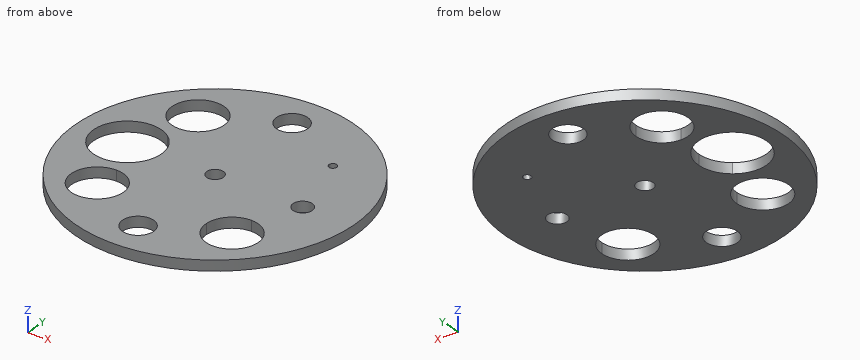
```python
from build123d import *

# Parameters (mm, degrees)
F0_R     = 26.75
F0_R_2   = 3
F0_R_3   = 1.85
F0_R_4   = 1.6
F1_DEPTH = 2


with BuildPart() as f1:
    # F0 (on Top) → F1 (new body)
    with BuildSketch(Plane.XY):
        Circle(F0_R)
        with Locations((0, -20)):
            Circle(F0_R_2, mode=Mode.SUBTRACT)
        with BuildLine():
            ThreePointArc((-13.081475, 8.081475), (-16.617009, 16.617009), (-8.081475, 13.081475))
            Line((-8.081475, 13.081475), (12.331475, 13.081475))
            ThreePointArc((12.331475, 13.081475), (13.081475, 13.831475), (13.831475, 13.081475))
            ThreePointArc((13.831475, 13.081475), (13.611806, 12.551145), (13.081475, 12.331475))
            Line((13.081475, 12.331475), (13.081475, -8.081475))
            ThreePointArc((13.081475, -8.081475), (16.617009, -9.545942), (18.081475, -13.081475))
            ThreePointArc((18.081475, -13.081475), (13.081475, -18.081475), (8.081475, -13.081475))
            Line((8.081475, -13.081475), (-8.081475, -13.081475))
            ThreePointArc((-8.081475, -13.081475), (-16.617009, -16.617009), (-13.081475, -8.081475))
            Line((-13.081475, -8.081475), (-13.081475, -5.186055))
            ThreePointArc((-13.081475, -5.186055), (-23.5, 0), (-13.081475, 5.186055))
            Line((-13.081475, 5.186055), (-13.081475, 8.081475))
        make_face(mode=Mode.SUBTRACT)
        with Locations((17, 0)):
            Circle(F0_R_3, mode=Mode.SUBTRACT)
        with Locations((0, 20)):
            Circle(F0_R_2, mode=Mode.SUBTRACT)
        with BuildLine():
            Line((12.331475, 13.081475), (-8.081475, 13.081475))
            ThreePointArc((-8.081475, 13.081475), (-9.545942, 9.545942), (-13.081475, 8.081475))
            Line((-13.081475, 8.081475), (-13.081475, 5.186055))
            ThreePointArc((-13.081475, 5.186055), (-11.181048, 2.896514), (-10.5, 0))
            ThreePointArc((-10.5, 0), (-11.181048, -2.896514), (-13.081475, -5.186055))
            Line((-13.081475, -5.186055), (-13.081475, -8.081475))
            ThreePointArc((-13.081475, -8.081475), (-9.545942, -9.545942), (-8.081475, -13.081475))
            Line((-8.081475, -13.081475), (8.081475, -13.081475))
            ThreePointArc((8.081475, -13.081475), (9.545942, -9.545942), (13.081475, -8.081475))
            Line((13.081475, -8.081475), (13.081475, 12.331475))
            ThreePointArc((13.081475, 12.331475), (12.551145, 12.551145), (12.331475, 13.081475))
        make_face()
        Circle(F0_R_4, mode=Mode.SUBTRACT)
    extrude(amount=F1_DEPTH)


solid = f1.part
```
Part model, mm, in its own coordinate system. Round coordinates to 2 decimals unless told otherwise and drop trailing zeros. Loops run counter-clockwise (first coordinate to the right, second up) from the corner with the lowest first, then second, coordinate; pieces in that order, holes last. Notation, with made-up numbers: (54.25, 20) -> (72.25, 20) arc R16 ccw to (72.25, 36) -> close; hole circle Ø1 at (-35, 47). An arc over 180 degrees is marked (long way). Use a Markdown table: item, result.
1) Probe line 1 (Y direction, x = 0, z = 1.1); line 2 (Y direction, x = 0.5, z = 0.9); line 3 (X direction, y = -9.5, z = 1.55). List the from-to ranges inside material, lowest first. Write a range as [from, to].
The answers:
| item | result |
|---|---|
| line 1 | y = [-26.75, -23], [-17, -1.6], [1.6, 17], [23, 26.75] |
| line 2 | y = [-26.75, -22.96], [-17.04, -1.52], [1.52, 17.04], [22.96, 26.75] |
| line 3 | x = [-25.01, -16.57], [-9.59, 9.59], [16.57, 25.01] |
2) Cut at C-C, the plane y = -11.5. List the corners of the cut face in (x, z).
The answers:
| item | result |
|---|---|
| outline | (-24.15, 0) -> (-17.82, 0) -> (-17.82, 2) -> (-24.15, 2) -> close; (-8.34, 0) -> (8.34, 0) -> (8.34, 2) -> (-8.34, 2) -> close; (17.82, 0) -> (24.15, 0) -> (24.15, 2) -> (17.82, 2) -> close |
3) Drop flat-ended pins along their axis: pin 1 Ø3 at (x, y) = (0, 0) entering from -Z; pin 2 Ø1 at (y, z) = (-21, 0.5) entering from +X. Give the stop position or say it passes through.
The answers:
| item | result |
|---|---|
| pin 1 | passes through |
| pin 2 | stops at x = 17.18 |
4) Cut at D-D, the plane y = 20. List the corners of the cut face in (x, z), and give its area (3 significant figures).
The answers:
| item | result |
|---|---|
| outline | (-17.76, 0) -> (-3, 0) -> (-3, 2) -> (-17.76, 2) -> close; (3, 0) -> (17.76, 0) -> (17.76, 2) -> (3, 2) -> close |
| area | 59.1 mm2 |
5) Cut at B-B, the plane z = 0.7. State how many separate pieces and enclosed holes the cut face has, and give its area (3 significant figures).
The answers:
| item | result |
|---|---|
| separate pieces | 1 |
| enclosed holes | 9 |
| area | 1,800 mm2 |
6) Cut at A-A, the plane x = 0. List the corners of the cut face in (y, z), and give its area (3 significant figures).
The answers:
| item | result |
|---|---|
| outline | (-26.75, 0) -> (-23, 0) -> (-23, 2) -> (-26.75, 2) -> close; (-17, 0) -> (-1.6, 0) -> (-1.6, 2) -> (-17, 2) -> close; (1.6, 0) -> (17, 0) -> (17, 2) -> (1.6, 2) -> close; (23, 0) -> (26.75, 0) -> (26.75, 2) -> (23, 2) -> close |
| area | 76.6 mm2 |
